```python
from build123d import *

# Parameters (mm, degrees)
CYLINDER001_R     = 2
CYLINDER001_DEPTH = 10
CYLINDER_R        = 2
CYLINDER_DEPTH    = 10
BOX_W             = 10
BOX_H             = 55
BOX_DEPTH         = 3
FILLET_R          = 2


with BuildPart() as h_bolt_l:
    # Cylinder001 → Cylinder001 (new body)
    with BuildSketch(Plane(origin=(5, 10, -4), x_dir=(1, 0, 0), z_dir=(0, 0, 1))):
        Circle(CYLINDER001_R)
    extrude(amount=CYLINDER001_DEPTH)


with BuildPart() as fusion:
    # Cylinder → Cylinder (new body)
    with BuildSketch(Plane(origin=(5, 48.5, -4), x_dir=(1, 0, 0), z_dir=(0, 0, 1))):
        Circle(CYLINDER_R)
    extrude(amount=CYLINDER_DEPTH)

    # Fusion: union h_bolt_l
    add(h_bolt_l.part)


with BuildPart() as fillet_body:
    # Box → Box (new body)
    with BuildSketch(Plane.XY):
        with Locations((5, 27.5)):
            Rectangle(BOX_W, BOX_H)
    extrude(amount=BOX_DEPTH)

    # Cut: cut Fusion
    add(fusion.part, mode=Mode.SUBTRACT)

    # Fillet
    fillet_edges = [fillet_body.edges().sort_by_distance(p)[0] for p in [
        (0, 0, 1.5),
        (0, 55, 1.5),
        (10, 0, 1.5),
        (10, 55, 1.5),
    ]]
    fillet(fillet_edges, radius=FILLET_R)


solid = fillet_body.part
```
Could you check a few things on this model? Use its own coordinates, in mm. Coordinates: 2 decimals unless noted, no trailing zeros. Loops run counter-clockwise (first coordinate to the right, second up) from the corner with the lowest first, then second, coordinate; pieces in that order, holes last.
1) Thinking about a two-plate mould opening in Y: for faces 1 (the face through (5, 0, 1)), 2 (the face through (10, 27, 1)), 3 (the face through (3.526, 11.352, 1.479)), which applies, released by +Y, released by -Y, zero draft, split by the parting line, or undercut?
Reported:
face 1: released by -Y
face 2: zero draft
face 3: undercut
2) Imagine slicing it at C-C (z = 0.65). List the corners of the cut face in (x, y) for me, and give its area (3 significant figures).
Reported:
outline: (0, 2) arc R2 ccw to (2, 0) - (8, 0) arc R2 ccw to (10, 2) - (10, 53) arc R2 ccw to (8, 55) - (2, 55) arc R2 ccw to (0, 53) - close; hole circle Ø4 at (5, 10); hole circle Ø4 at (5, 48.5)
area: 521 mm2
3) Imagine slicing it at A-A (x = 5). List the corners of the cut face in (y, z) for me, and give its area (3 significant figures).
Reported:
outline: (0, 0) - (8, 0) - (8, 3) - (0, 3) - close; (12, 0) - (46.5, 0) - (46.5, 3) - (12, 3) - close; (50.5, 0) - (55, 0) - (55, 3) - (50.5, 3) - close
area: 141 mm2
4) Will this pin go through, and if not, where does the flat tip stop? pin 1 Ø2.5 at (x, y) = (5, 10) entering from +Z.
Reported:
pin 1: passes through
5) Please list where these lines run through material, in increasing order: line 1 along Y through (x, z) = (5, 1); line 2 along X through (y, z) = (48.5, 1.3); line 3 along X through (y, z) = (9, 1.3).
Reported:
line 1: y = 0 to 8, 12 to 46.5, 50.5 to 55
line 2: x = 0 to 3, 7 to 10
line 3: x = 0 to 3.27, 6.73 to 10
6) Imagine slicing it at B-B (y = 10). List the corners of the cut face in (x, z) for me.
Reported:
outline: (0, 0) - (3, 0) - (3, 3) - (0, 3) - close; (7, 0) - (10, 0) - (10, 3) - (7, 3) - close
